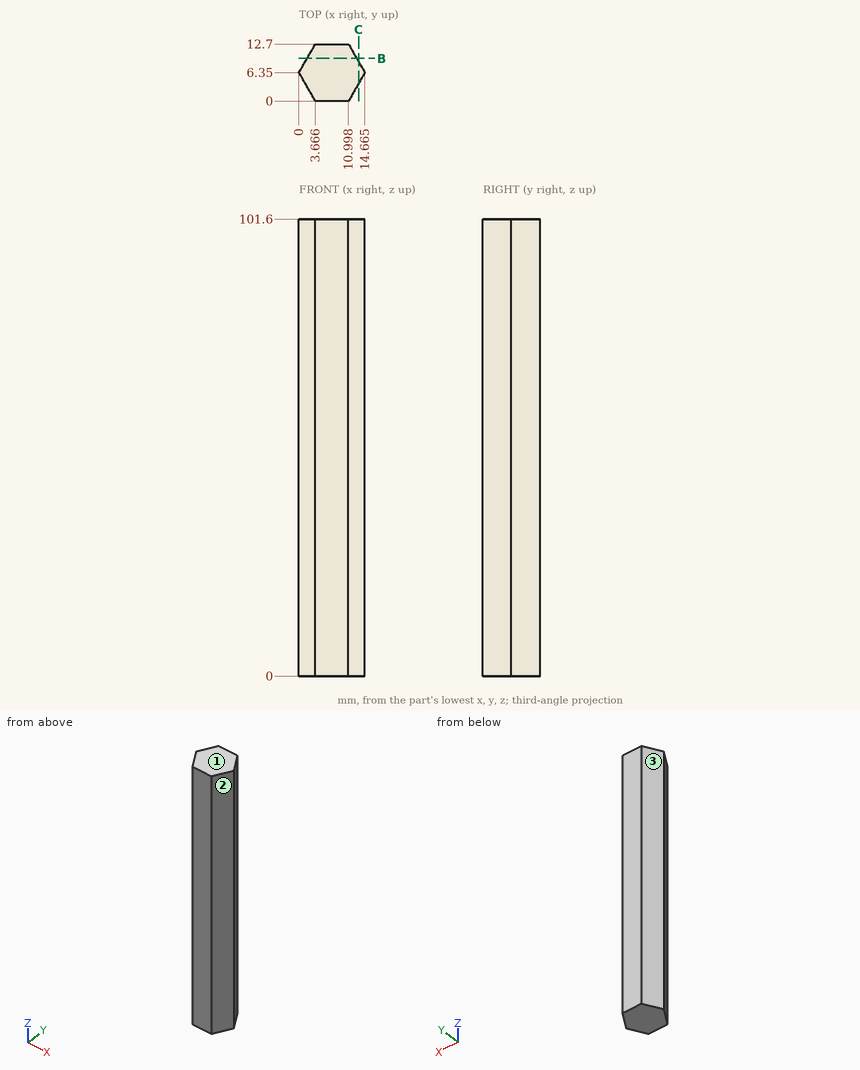
Part print with two shaded views. Sizes in mm from the minimum x, y, z corner. Give positions to 0.01 mm unless a question says otherwise; leave off trailing zeros. Order: outer loops, then holes, each group sorted by start corner. A loop starts at its lowest first (then second) coordinate and runs counter-clockwise, first axis right, second up.
1) Mould opens along Y. For the marked faces 1, 2 and 3 say: +Y half, -Y half, draft (parallel to the pull), parting line (faces both ways), or undercut.
2) Pin check, flat tips, straight feed: pin 1 (2 mm diameter, centred on y = 10.5, z = 30, fed in from +X) (1 decimal); pin 2 (6 mm diameter, centred on x = 11.5, y = 3, fed in from -Z); pin 3 (1.5 mm diameter, centred on y = 5, z = 15, fed in from +X). Stop position of each tip, or through.
3) Saw through at C-C, the plane x = 13.25. Write the cut outline in (y, z), then the cut area to 3 significant figures.
4) Saw through at B-B, the plane y = 9.5. Write the cut outline in (x, z) (1 decimal), then the cut area to 3 significant figures.
5) Wall check: probe 1 along Y at (x, z) = (1, 53) (1 decimal); probe 2 along Y at (x, z) = (2.5, 70); probe 3 along X at (y, z) = (6, 48). Give the ranges that are in metal, low to high.
Computed:
1. face 1: draft
1. face 2: -Y half
1. face 3: +Y half
2. pin 1: stops at x = 12.8
2. pin 2: stops at z = 0
2. pin 3: stops at x = 14.32
3. outline: (3.9, 0) - (8.8, 0) - (8.8, 101.6) - (3.9, 101.6) - close
3. area: 498 mm2
4. outline: (1.8, 0) - (12.8, 0) - (12.8, 101.6) - (1.8, 101.6) - close
4. area: 1,120 mm2
5. probe 1: y = 4.6 to 8.1
5. probe 2: y = 2.02 to 10.68
5. probe 3: x = 0.2 to 14.46
